The listing builds one solid part. Answer for the finished solid, in the listing's coordinates (mm). Face numbers are marked on the shaded views. A direction names the side the tool comes from. Give positions to 0.01 mm unless a question says otherwise; leave off trailing zeros. Write each loop counter-clockwise with the first axis right and the second up, starting at its lowest first coordinate (ties: lowest second). Pieces come first, ordered by that corner, then holes. Notation, with made-up numbers: (60.5, -16.75) - (78.5, -16.75) arc R9 ccw to (78.5, -8.75) - close; hole circle Ø10 at (73.5, -35). An arc over 180 degrees is marked (long way). One line per item, written item: value. Start each with the question number.
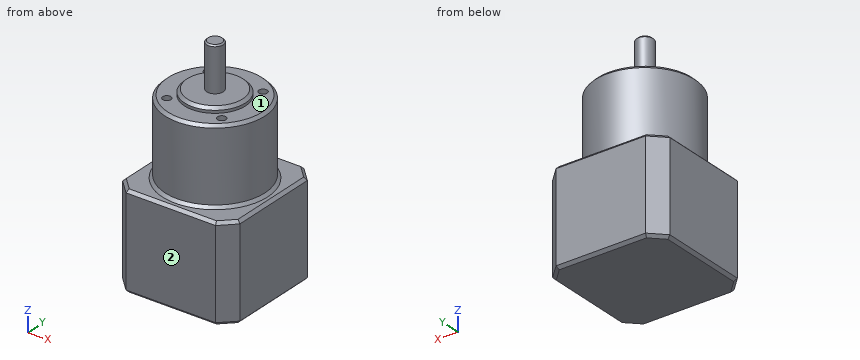
from build123d import *

# Parameters (mm, degrees)
SKETCH1_W           = 42.3
SKETCH1_H           = 42.3
BOSS_EXTRUDE1_DEPTH = 34
CHAMFER1_SIZE       = 5
SKETCH2_R           = 18
BOSS_EXTRUDE2_DEPTH = 27.3
SKETCH3_R           = 11
BOSS_EXTRUDE3_DEPTH = 2
SKETCH4_R           = 3
BOSS_EXTRUDE4_DEPTH = 16
CHAMFER2_SIZE       = 1
CHAMFER3_SIZE       = 0.5
SKETCH5_R           = 1.5
CUT_EXTRUDE1_DEPTH  = 5
ECHELLE1_SCALE      = 2
ECHELLE2_SCALE      = 0.25


with BuildPart() as part:
    # Sketch1 → Boss-Extrude1 (new body)
    with BuildSketch(Plane.XY):
        Rectangle(SKETCH1_W, SKETCH1_H)
    extrude(amount=BOSS_EXTRUDE1_DEPTH)

    # Chamfer1
    chamfer1_edges = [part.edges().sort_by_distance(p)[0] for p in [
        (21.15, -21.15, 17),
        (-21.15, -21.15, 17),
        (-21.15, 21.15, 17),
        (21.15, 21.15, 17),
    ]]
    chamfer(chamfer1_edges, length=CHAMFER1_SIZE)

    # Sketch2 → Boss-Extrude2 (add)
    with BuildSketch(Plane.XY.offset(34)):
        Circle(SKETCH2_R)
    extrude(amount=BOSS_EXTRUDE2_DEPTH)

    # Sketch3 → Boss-Extrude3 (add)
    with BuildSketch(Plane.XY.offset(61.3)):
        Circle(SKETCH3_R)
    extrude(amount=BOSS_EXTRUDE3_DEPTH)

    # Sketch4 → Boss-Extrude4 (add)
    with BuildSketch(Plane.XY.offset(63.3)):
        Circle(SKETCH4_R)
    extrude(amount=BOSS_EXTRUDE4_DEPTH)

    # Chamfer2
    chamfer2_edges = [part.edges().sort_by_distance(p)[0] for p in [
        (0, -21.15, 0),
        (0, -21.15, 34),
        (21.15, 0, 0),
        (-21.15, 0, 0),
        (0, 21.15, 0),
        (18.65, 18.65, 0),
        (18.65, -18.65, 0),
        (-18.65, 18.65, 0),
        (-18.65, -18.65, 0),
        (-21.15, 0, 34),
        (21.15, 0, 34),
        (0, 21.15, 34),
        (18.65, 18.65, 34),
        (18.65, -18.65, 34),
        (-18.65, 18.65, 34),
        (-18.65, -18.65, 34),
        (-18, 0, 34),
        (-18, 0, 61.3),
        (-11, 0, 63.3),
    ]]
    chamfer(chamfer2_edges, length=CHAMFER2_SIZE)

    # Chamfer3
    chamfer3_edges = [part.edges().sort_by_distance(p)[0] for p in [
        (-3, 0, 79.3),
    ]]
    chamfer(chamfer3_edges, length=CHAMFER3_SIZE)

    # Sketch5 → Cut-Extrude1 (cut)
    with BuildSketch(Plane.XY.offset(61.3)):
        with Locations((9.899494937, 9.899494937)):
            Circle(SKETCH5_R)
        with Locations((9.899494937, -9.899494937)):
            Circle(SKETCH5_R)
        with Locations((-9.899494937, -9.899494937)):
            Circle(SKETCH5_R)
        with Locations((-9.899494937, 9.899494937)):
            Circle(SKETCH5_R)
    extrude(amount=-CUT_EXTRUDE1_DEPTH, mode=Mode.SUBTRACT)


with BuildPart() as part_1:
    # Echelle1: scaled about (0, 0, 27.268947418)
    add(part.part.scale(ECHELLE1_SCALE).moved(Location((0, 0, -27.268947418))))


with BuildPart() as part_2:
    # Echelle2: scaled about (0, 0, 27.268947418)
    add(part_1.part.scale(ECHELLE2_SCALE).moved(Location((0, 0, 20.451710564))))


solid = part_2.part
Item 1: Find section B-B on z = 18.5. Determine the outline of the cut face in (x, y) (3 decimals), plus the area to 3 significant figures.
Item 2: For the marked faces 1 and 2, determine the directions among +Z, -Z, +X, -X, +Y, -Y from which every point of the face is accessible in a straight line to the end or side of a thin tool.
Item 3: Find section D-D on z = 50.5. Determine the outline of the cut face in (x, y), plus the area to 3 significant figures.
Item 4: Straight lines are drawn through the part: line 1 along Y through (x, z) = (5.5, 42); line 2 along Z through (x, y) = (5.5, 9.25); line 3 along Z through (x, y) = (3.25, -4.5). For each, find the intervals that lie inside material, in ascending order.
Item 5: Find section A-A on y = 0. Determine the outline of the cut face in (x, z) (3 decimals).
Item 6: Each of these flat-tipped pins is pushed along its axis until it touches: pin 1 Ø10 at (x, z) = (7.5, 37.5) entering from -Y; pin 2 Ø8 at (x, y) = (1, -1.5) entering from +Z; pin 3 Ø8 at (y, z) = (4, 37) entering from -X; pin 4 Ø0.8 at (x, y) = (4.5, 5) entering from +Z. Where does it stop, or does it pass through?
Values:
1. outline: (-10.575, -8.075) - (-8.075, -10.575) - (8.075, -10.575) - (10.575, -8.075) - (10.575, 8.075) - (8.075, 10.575) - (-8.075, 10.575) - (-10.575, 8.075) - close
1. area: 435 mm^2
2. face 1: +Z
2. face 2: +Z, -Z, +X, -X, -Y
3. outline: circle Ø3 at (0, 0)
3. area: 7.07 mm^2
4. line 1: -7.12 to -5.46, -4.44 to 4.44, 5.46 to 7.12
4. line 2: 13.63 to 30.63
4. line 3: 13.63 to 44.28
5. outline: (-10.575, 14.134) - (-10.075, 13.634) - (10.075, 13.634) - (10.575, 14.134) - (10.575, 30.134) - (10.075, 30.634) - (9.5, 30.634) - (9, 31.134) - (9, 43.784) - (8.5, 44.284) - (5.5, 44.284) - (5.5, 44.784) - (5, 45.284) - (1.5, 45.284) - (1.5, 53.034) - (1.25, 53.284) - (-1.25, 53.284) - (-1.5, 53.034) - (-1.5, 45.284) - (-5, 45.284) - (-5.5, 44.784) - (-5.5, 44.284) - (-8.5, 44.284) - (-9, 43.784) - (-9, 31.134) - (-9.5, 30.634) - (-10.075, 30.634) - (-10.575, 30.134) - close
6. pin 1: y = -8.65
6. pin 2: z = 53.28
6. pin 3: x = -9
6. pin 4: z = 44.28
